Drawing for the job (mm, zero at the part's lowest x, y, z). A direction names the side the tool comes from. Round coordinates to 2 decimals unless told otherwise and drop trailing zeros. Write each loop counter-clockwise with the first axis right and the second up, starting at its lowest first coordinate (ties: lowest second). Pieces come first, ordered by that corner, then holes. Notation, with made-up numbers: (-2.75, 89) - (4.25, 89) arc R29 cw to (4.25, 115) - close; hole circle Ø6 at (12, -33). An arc over 180 degrees is marked (long way). Answer in a Markdown table with one row per item.
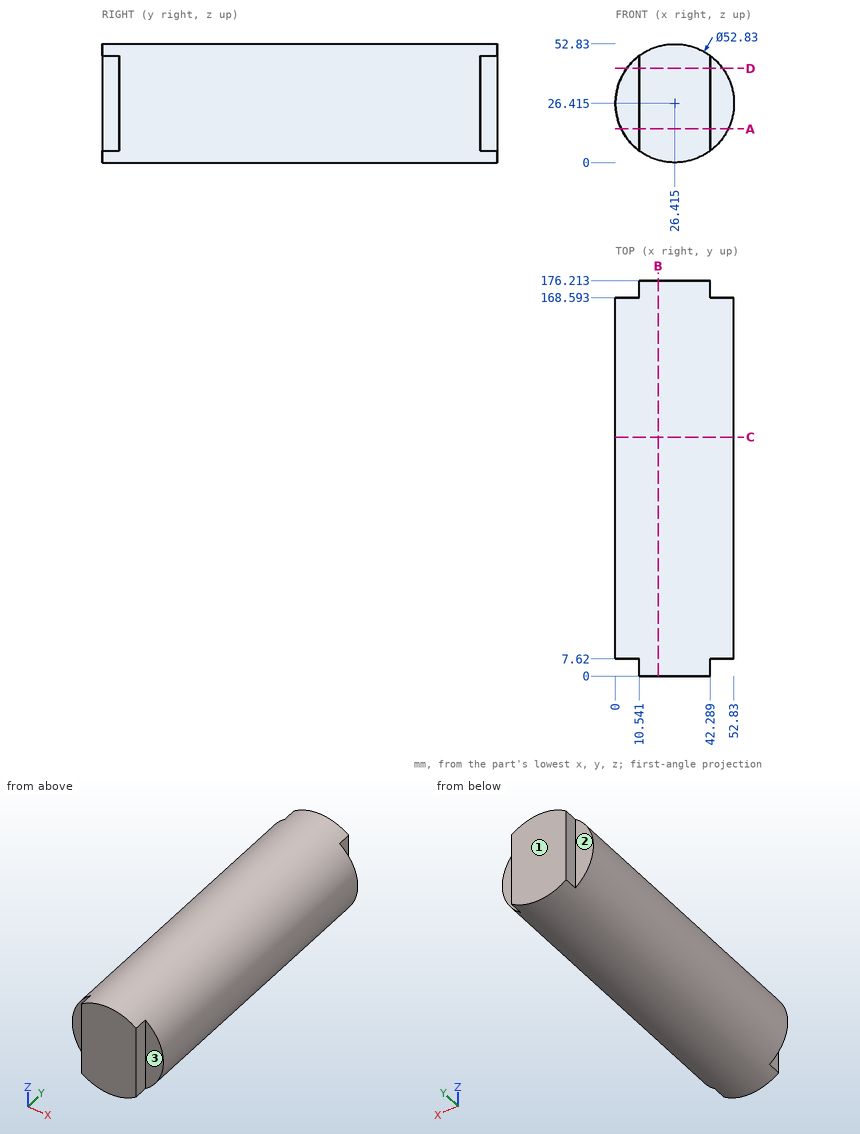
Q1. Drill centre lines: line 1 (Y direction, x = 4, z = 29); line 2 (Z direction, x = 25.5, y = 17.5) (1 decimal); line 3 (X direction, y = 65, z = 47.5) (1 decimal). Where is each one in solid material? Low to high.
Computed:
| item | result |
|---|---|
| line 1 | y = 7.62 to 168.59 |
| line 2 | z = 0 to 52.8 |
| line 3 | x = 10.5 to 42.3 |
Q2. Saw through at C-C on y = 106.5. List the corners of the cut face in (x, z) (1 decimal).
Computed:
| item | result |
|---|---|
| outline | circle Ø52.8 at (26.4, 26.4) |
Q3. Saw through at B-B on x = 19. List the corners of the cut face in (y, z), then the cut area to 4 significant figures.
Computed:
| item | result |
|---|---|
| outline | (0, 1.06) - (176.21, 1.06) - (176.21, 51.77) - (0, 51.77) - close |
| area | 8,935 mm2 |
Q4. 3-axis set-ups, long thin cutter, end or side, ignore diameter. For the marked faces 1, 2 and 3: which of +Z, -Z, +X, -X, +Y, -Y reach the whole face in a straight line?
Computed:
| item | result |
|---|---|
| face 1 | +Z, -Z, +X, -X, +Y |
| face 2 | +Z, -Z, -X, +Y |
| face 3 | +Z, -Z, +X, -Y |
Q5. Saw through at D-D on z = 42. List the corners of the cut face in (x, y).
Computed:
| item | result |
|---|---|
| outline | (5.09, 7.62) - (10.54, 7.62) - (10.54, 0) - (42.29, 0) - (42.29, 7.62) - (47.74, 7.62) - (47.74, 168.59) - (42.29, 168.59) - (42.29, 176.21) - (10.54, 176.21) - (10.54, 168.59) - (5.09, 168.59) - close |
Q6. Flat gauge pins, fed straight in: pin 1 (5 mm diameter, centred on y = 55, z = 11.5, fed in from -X); pin 2 (4 mm diameter, centred on y = 3, z = 31, fed in from -X); pin 3 (1.5 mm diameter, centred on x = 47, z = 46, fed in from -Y); pin 4 (8.5 mm diameter, centred on y = 2, z = 31.5, fed in from +X). Where does each tip first touch, or does it go through?
Computed:
| item | result |
|---|---|
| pin 1 | stops at x = 3.1 |
| pin 2 | stops at x = 10.54 |
| pin 3 | passes through |
| pin 4 | stops at x = 42.29 |
Q7. Saw through at A-A on z = 15. List the corners of the cut face in (x, y).
Computed:
| item | result |
|---|---|
| outline | (2.59, 7.62) - (10.54, 7.62) - (10.54, 0) - (42.29, 0) - (42.29, 7.62) - (50.24, 7.62) - (50.24, 168.59) - (42.29, 168.59) - (42.29, 176.21) - (10.54, 176.21) - (10.54, 168.59) - (2.59, 168.59) - close |
